For this review, take the finished solid that the model builds, in its own axes (mm). A direction names the side the tool comes from. Coordinates: 2 decimals unless noted, no trailing zeros. Loops run counter-clockwise (first coordinate to the right, second up) from the corner with the lowest first, then second, coordinate; pieces in that order, holes last. Notation, with made-up numbers: (31.25, -18) -> (54.25, -18) arc R28 cw to (54.25, 19) -> close; hole circle Ø10 at (-4, -1). An arc over 180 degrees is marked (long way). Use a Markdown table: item, result.
from build123d import *

# Parameters (mm, degrees)
BOSS_EXTRUDE1_DEPTH = 40
SKETCH2_R           = 4
CUT_EXTRUDE1_DEPTH  = 40
CUT_EXTRUDE2_REACH  = 97.306
CUT_EXTRUDE3_REACH  = 91.766
SKETCH4_R           = 4


with BuildPart() as part:
    # Sketch1 → Boss-Extrude1 (new body)
    with BuildSketch(Plane.XY):
        with BuildLine():
            Line((0, 5), (0, 0))
            Line((0, 0), (37.113248654, 0))
            ThreePointArc((37.113248654, 0), (39.613248654, 0.669872981), (41.443375673, 2.5))
            Line((41.443375673, 2.5), (62.5, 38.97114317))
            ThreePointArc((62.5, 38.97114317), (65.536031793, 41.300772302), (69.330127019, 40.801270189))
            Line((69.330127019, 40.801270189), (82.320508076, 33.301270189))
            Line((82.320508076, 33.301270189), (84.820508076, 37.631397208))
            Line((84.820508076, 37.631397208), (67.5, 47.631397208))
            ThreePointArc((67.5, 47.631397208), (63.705904774, 48.130899321), (60.669872981, 45.801270189))
            Line((60.669872981, 45.801270189), (38.556624327, 7.5))
            ThreePointArc((38.556624327, 7.5), (36.726497308, 5.669872981), (34.226497308, 5))
            Line((34.226497308, 5), (0, 5))
        make_face()
    extrude(amount=BOSS_EXTRUDE1_DEPTH)

    # Sketch2 → Cut-Extrude1 (cut)
    with BuildSketch(Plane(origin=(0, 5, 0), x_dir=(1, 0, 0), z_dir=(0, 1, 0))):
        with Locations(Location((12, -12, 0), (0, 0, 270))):
            Circle(SKETCH2_R)
        with Locations(Location((12, -28, 0), (0, 0, 270))):
            Circle(SKETCH2_R)
    extrude(amount=-CUT_EXTRUDE1_DEPTH, mode=Mode.SUBTRACT)

    # Sketch3 → Cut-Extrude2 (cut, up to next)
    with BuildSketch(Plane(origin=(25.669872981, -14.820508076, 0), x_dir=(0, 0, 1), z_dir=(-0.86602540378444, 0.49999999999999784, 0)), mode=Mode.PRIVATE) as cut_extrude2_sk1:
        with BuildLine():
            Line((19, 48), (0, 48))
            Line((0, 48), (0, 42))
            Line((0, 42), (19, 42))
            ThreePointArc((19, 42), (22, 45), (19, 48))
        make_face()
    cut_extrude2_tool1 = extrude(cut_extrude2_sk1.sketch, amount=-CUT_EXTRUDE2_REACH, mode=Mode.PRIVATE) & part.part
    add(cut_extrude2_tool1.solids().sort_by_distance((48.169873, 24.150635, 10.688594))[0], mode=Mode.SUBTRACT)

    # Sketch4 → Cut-Extrude3 (cut, up to next)
    with BuildSketch(Plane(origin=(37.5, 64.951905284, 0), x_dir=(0.8660254037844429, -0.49999999999999284, 0), z_dir=(0.49999999999999284, 0.8660254037844429, 0)), mode=Mode.PRIVATE) as cut_extrude3_sk1:
        with Locations(Location((44.641016151, -28, 0), (0, 0, 180))):
            Circle(SKETCH4_R)
    cut_extrude3_tool1 = extrude(cut_extrude3_sk1.sketch, amount=-CUT_EXTRUDE3_REACH, mode=Mode.PRIVATE) & part.part
    # Sketch4 → Cut-Extrude3 (cut, up to next)
    with BuildSketch(Plane(origin=(37.5, 64.951905284, 0), x_dir=(0.8660254037844429, -0.49999999999999284, 0), z_dir=(0.49999999999999284, 0.8660254037844429, 0)), mode=Mode.PRIVATE) as cut_extrude3_sk2:
        with Locations(Location((44.641016151, -12, 0), (0, 0, 180))):
            Circle(SKETCH4_R)
    cut_extrude3_tool2 = extrude(cut_extrude3_sk2.sketch, amount=-CUT_EXTRUDE3_REACH, mode=Mode.PRIVATE) & part.part
    add(cut_extrude3_tool1.solids().sort_by_distance((76.160254, 42.631397, 28))[0], mode=Mode.SUBTRACT)
    add(cut_extrude3_tool2.solids().sort_by_distance((76.160254, 42.631397, 12))[0], mode=Mode.SUBTRACT)


solid = part.part
(1) For pin 1 Ø4 at (y, z) = (25.5, 9.5) entering from +X; pin 2 Ø3 at (y, z) = (26.5, 14.5) entering from -X; pin 3 Ø13 at (x, z) = (12, 28) entering from +Y; pin 4 Ø6.5 at (x, z) = (12, 12) entering from -Y, all flat-tipped, find the tip position at first contact; note any pin that passes through.
Found:
| item | result |
|---|---|
| pin 1 | stops at x = 55.88 |
| pin 2 | stops at x = 49.67 |
| pin 3 | stops at y = 5 |
| pin 4 | passes through |
(2) For line 1 along Y through (x, z) = (27, 9); line 2 along X through (y, z) = (1.7, 12); line 3 along X through (y, z) = (2.4, 12), list the stretches that pass through material, from the lowest coordinate up.
Found:
| item | result |
|---|---|
| line 1 | y = 0 to 5 |
| line 2 | x = 0 to 8, 16 to 40.87 |
| line 3 | x = 0 to 8, 16 to 41.38 |
(3) Mouldability with a two-part tool opening along Y and no side actions: class faces 1 (the face through (49.77, 26.92, 19.72)), 2 (the face through (50, 23, 22)), 3 (the face through (0, 3, 20)) as pulls with the +Y half, pulls with the -Y half, needs draft (parallel to the pull), parting line crosses it, or undercut.
Found:
| item | result |
|---|---|
| face 1 | pulls with the +Y half |
| face 2 | undercut |
| face 3 | needs draft |
(4) Take a section at C-C on z = 10. Write out the cut boundary in (x, y), plus the area to 3 significant figures.
Found:
| item | result |
|---|---|
| outline | (0, 0) -> (8.54, 0) -> (8.54, 5) -> (0, 5) -> close; (15.46, 0) -> (37.11, 0) arc R5 ccw to (41.44, 2.5) -> (51, 19.05) -> (46.67, 21.55) -> (38.56, 7.5) arc R5 cw to (34.23, 5) -> (15.46, 5) -> close; (49.67, 26.75) -> (54, 24.25) -> (62.5, 38.97) arc R5 cw to (69.33, 40.8) -> (70.66, 40.03) -> (73.16, 44.36) -> (67.5, 47.63) arc R5 ccw to (60.67, 45.8) -> close; (76.66, 36.57) -> (82.32, 33.3) -> (84.82, 37.63) -> (79.16, 40.9) -> close |
| area | 461 mm^2 |
(5) Take a section at A-A on x = 12. Write out the cut boundary in (y, z).
Found:
| item | result |
|---|---|
| outline | (0, 0) -> (5, 0) -> (5, 8) -> (0, 8) -> close; (0, 16) -> (5, 16) -> (5, 24) -> (0, 24) -> close; (0, 32) -> (5, 32) -> (5, 40) -> (0, 40) -> close |
(6) Take a section at D-D on z = 28. Write out the cut boundary in (x, y), plus the area to 3 significant figures.
Found:
| item | result |
|---|---|
| outline | (0, 0) -> (8, 0) -> (8, 5) -> (0, 5) -> close; (16, 0) -> (37.11, 0) arc R5 ccw to (41.44, 2.5) -> (62.5, 38.97) arc R5 cw to (69.33, 40.8) -> (70.2, 40.3) -> (72.7, 44.63) -> (67.5, 47.63) arc R5 ccw to (60.67, 45.8) -> (38.56, 7.5) arc R5 cw to (34.23, 5) -> (16, 5) -> close; (77.12, 36.3) -> (82.32, 33.3) -> (84.82, 37.63) -> (79.62, 40.63) -> close |
| area | 481 mm^2 |
(7) Take a section at B-B on z = 5. Write out the cut boundary in (x, y), plus the area to 3 significant figures.
Found:
| item | result |
|---|---|
| outline | (0, 0) -> (37.11, 0) arc R5 ccw to (41.44, 2.5) -> (51, 19.05) -> (46.67, 21.55) -> (38.56, 7.5) arc R5 cw to (34.23, 5) -> (0, 5) -> close; (49.67, 26.75) -> (54, 24.25) -> (62.5, 38.97) arc R5 cw to (69.33, 40.8) -> (82.32, 33.3) -> (84.82, 37.63) -> (67.5, 47.63) arc R5 ccw to (60.67, 45.8) -> close |
| area | 531 mm^2 |
(8) For faces 4 (the face through (17, 5, 20)), 5 (the face through (75.734, 37.104, 19.72)), 6 (the face through (48.805, 20.32, 9.367)), list the 3-axis set-ups (+Z, -Z, +X, -X, +Y, -Y) from which the entire face can be reached by the end or side of a thin tool; tool diameter is ignored.
Found:
| item | result |
|---|---|
| face 4 | +Z, -Z, -X, +Y |
| face 5 | +Z, -Z, -Y |
| face 6 | -Z, +X |
